from build123d import *

# Parameters (mm, degrees)
SKETCH3_W               = 100
SKETCH3_H               = 210
BOSS_EXTRUDE2_DEPTH     = 5
SKETCH2_W               = 4.8
SKETCH2_H               = 15.2
SKETCH2_W_2             = 5.2
CORTAR_EXTRUIR1_DEPTH   = 2
FILLET1_R               = 2
CUT_EXTRUDE1_DEPTH      = 233.647802483
CUT_EXTRUDE1_DEPTH_BACK = 233.647802483
SKETCH6_R               = 1
CUT_EXTRUDE2_DEPTH      = 3
SKETCH6_4_R             = 1.5
AGUJEROSL298N_DEPTH     = 233.647802483
SKETCH6_6_W             = 68
SKETCH6_6_H             = 35
SKETCH6_6_W_2           = 43
SKETCH6_6_H_2           = 43
SKETCH6_6_H_3           = 20.6
CORTAR_EXTRUIR2_DEPTH   = 2


with BuildPart() as part:
    # Sketch3 → Boss-Extrude2 (new body)
    with BuildSketch(Plane(origin=(0, 0, 0), x_dir=(1, 0, 0), z_dir=(0, 1, 0))):
        with Locations((-50, 105)):
            Rectangle(SKETCH3_W, SKETCH3_H)
    extrude(amount=BOSS_EXTRUDE2_DEPTH)

    # Sketch2 → Cortar-Extruir1 (cut)
    with BuildSketch(Plane(origin=(0, 0, 0), x_dir=(-1, 0, 0), z_dir=(0, -1, 0))):
        with Locations((6, 172.3)):
            Rectangle(SKETCH2_W, SKETCH2_H)
        with Locations((94, 172.3)):
            Rectangle(SKETCH2_W_2, SKETCH2_H)
        with Locations((94, 37.7)):
            Rectangle(SKETCH2_W, SKETCH2_H)
        with Locations((6, 37.7)):
            Rectangle(SKETCH2_W, SKETCH2_H)
    extrude(amount=-CORTAR_EXTRUIR1_DEPTH, mode=Mode.SUBTRACT)

    # Fillet1
    fillet1_edges = [part.edges().sort_by_distance(p)[0] for p in [
        (0, 5, -105),
        (-50, 5, -210),
        (-100, 5, -105),
        (-50, 0, -210),
        (0, 0, -105),
        (-50, 0, 0),
        (-100, 0, -105),
        (-100, 2.5, -210),
        (0, 2.5, -210),
        (-50, 5, 0),
    ]]
    fillet(fillet1_edges, radius=FILLET1_R)

    # Sketch4 → Cut-Extrude1 (cut, two sides: drawn at the far end of the back side and taken through both)
    with BuildSketch(Plane(origin=(0, 5, 0), x_dir=(1, 0, 0), z_dir=(0, 1, 0)).offset(-CUT_EXTRUDE1_DEPTH_BACK)):
        with BuildLine():
            Line((-7.5, 110), (-7.5, 100))
            ThreePointArc((-7.5, 100), (-10, 97.5), (-12.5, 100))
            Line((-12.5, 100), (-12.5, 110))
            ThreePointArc((-12.5, 110), (-10, 112.5), (-7.5, 110))
        make_face()
        with BuildLine():
            Line((-92.5, 110), (-92.5, 100))
            ThreePointArc((-92.5, 100), (-90, 97.5), (-87.5, 100))
            Line((-87.5, 100), (-87.5, 110))
            ThreePointArc((-87.5, 110), (-90, 112.5), (-92.5, 110))
        make_face()
    extrude(amount=CUT_EXTRUDE1_DEPTH + CUT_EXTRUDE1_DEPTH_BACK, mode=Mode.SUBTRACT)

    # Sketch6 → Cut-Extrude2 (cut)
    with BuildSketch(Plane(origin=(0, 5, 0), x_dir=(1, 0, 0), z_dir=(0, 1, 0))):
        with Locations(Location((-80, 202, 0), (0, 0, 270))):
            Circle(SKETCH6_R)
        with Locations(Location((-20, 202, 0), (0, 0, 90))):
            Circle(SKETCH6_R)
        with Locations(Location((-20, 8, 0), (0, 0, 270))):
            Circle(SKETCH6_R)
        with Locations(Location((-80, 8, 0), (0, 0, 90))):
            Circle(SKETCH6_R)
    extrude(amount=-CUT_EXTRUDE2_DEPTH, mode=Mode.SUBTRACT)

    # Sketch6_4 → AgujerosL298N (cut, through all)
    with BuildSketch(Plane(origin=(0, 5, 0), x_dir=(1, 0, 0), z_dir=(0, 1, 0))):
        with Locations(Location((-30.5, 196, 0), (0, 0, 270))):
            Circle(SKETCH6_4_R)
        with Locations(Location((-69.5, 157, 0), (0, 0, 270))):
            Circle(SKETCH6_4_R)
        with Locations(Location((-30.5, 157, 0), (0, 0, 270))):
            Circle(SKETCH6_4_R)
        with Locations(Location((-69.5, 196, 0), (0, 0, 90))):
            Circle(SKETCH6_4_R)
    extrude(amount=-AGUJEROSL298N_DEPTH, mode=Mode.SUBTRACT)

    # Sketch6_6 → Cortar-Extruir2 (cut)
    with BuildSketch(Plane(origin=(0, 5, 0), x_dir=(1, 0, 0), z_dir=(0, 1, 0))):
        with Locations((-50, 29.5)):
            Rectangle(SKETCH6_6_W, SKETCH6_6_H)
        with Locations((-50, 176.5)):
            Rectangle(SKETCH6_6_W_2, SKETCH6_6_H_2)
        with Locations((-50, 70.922705979)):
            Rectangle(SKETCH6_6_W_2, SKETCH6_6_H_3)
        with Locations((-50, 97.904338996)):
            Rectangle(SKETCH6_6_W_2, SKETCH6_6_H_3)
    extrude(amount=-CORTAR_EXTRUIR2_DEPTH, mode=Mode.SUBTRACT)


solid = part.part
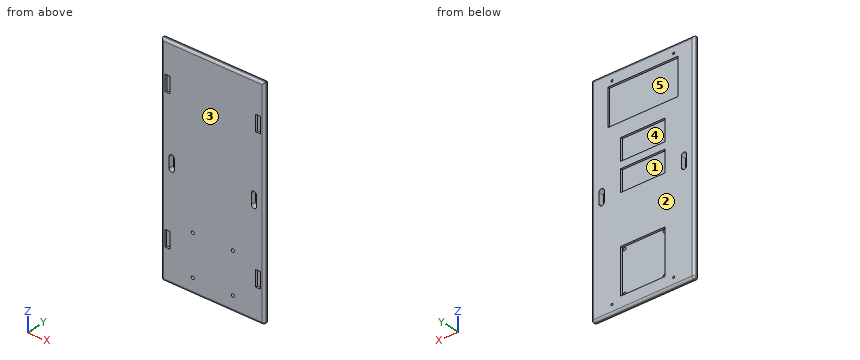
Model file for the job. Use its own axes, mm. Face numbers are marked on the shaded views. A direction names the side the tool comes from. Coordinates: 2 decimals unless noted, no trailing zeros. Write each loop counter-clockwise with the first axis right and the second up, starting at its lowest first coordinate (ties: lowest second). Pieces come first, ordered by that corner, then holes. Notation, with made-up numbers: (-20, -31) -> (-15, -31) arc R19 cw to (-15, -27) -> close; hole circle Ø10 at (-25, 55). An arc over 180 degrees is marked (long way). One line per item, written item: value. Start each with the question number.
1) Slice it at D-D on x = -25.5. Write the cut outline in (y, z), then the cut area to 3 significant figures.
2) Probe probe 1 along Z at (x, y) = (-80, 3.2); probe 2 along X at (y, z) = (2.75, -202); probe 3 along Z at (x, y) = (-69.5, 2.2). List the from-to ranges inside material, lowest first.
3) Flat gauge pins, fed straight in: pin 1 Ø1.8 at (x, z) = (-69.5, -196) entering from -Y; pin 2 Ø17.5 at (x, z) = (-37.5, -30) entering from +Y; pin 3 Ø1.6 at (x, y) = (-6, 1) entering from +Z; pin 4 Ø1 at (x, y) = (-6, 0.5) entering from -Z. Where does each tip first touch, or does it go through?
4) Slice it at B-B on x = -42. Write the cut outline in (y, z).
5) Which spindle directions (+Z, -Z, +X, -X, +Y, -Y) get a long thin tool onto all of the face, cutting with end or side? Do the marked faces 1 and 2. Say none if no direction does.
6) Slice it at C-C on z = -75.5. Write the cut outline in (x, y), then the cut area to 3 significant figures.
7) Slice it at A-A on z = -104.5. Write the cut outline in (x, y).
8) Pull direction X, two halves, no side cores. Call the marked faces 3, 4 and 5: +X half, -X half, draft (parallel to the pull), parting line (faces both ways), or undercut.
Answers follow:
1. outline: (0, -208) arc R2 ccw to (2, -210) -> (3, -210) arc R2 ccw to (5, -208) -> (5, -47) -> (3, -47) -> (3, -12) -> (5, -12) -> (5, -2) arc R2 ccw to (3, 0) -> (2, 0) arc R2 ccw to (0, -2) -> close
1. area: 977 mm2
2. probe 1: -209.99 to -203, -201 to -47, -12 to -9, -7 to -0.01
2. probe 2: -100 to -81, -79 to -21, -19 to 0
2. probe 3: -210 to -197.5, -194.5 to -158.5, -155.5 to 0
3. pin 1: through
3. pin 2: y = 3
3. pin 3: z = -0.01
3. pin 4: z = -209.73
4. outline: (0, -208) arc R2 ccw to (2, -210) -> (3, -210) arc R2 ccw to (5, -208) -> (5, -198) -> (3, -198) -> (3, -155) -> (5, -155) -> (5, -108.2) -> (3, -108.2) -> (3, -87.6) -> (5, -87.6) -> (5, -81.22) -> (3, -81.22) -> (3, -60.62) -> (5, -60.62) -> (5, -47) -> (3, -47) -> (3, -12) -> (5, -12) -> (5, -2) arc R2 ccw to (3, 0) -> (2, 0) arc R2 ccw to (0, -2) -> close
5. face 1: +Y
5. face 2: +Z, -Z, +X, -X, +Y
6. outline: (-100, 2) arc R2 ccw to (-98, 0) -> (-2, 0) arc R2 ccw to (0, 2) -> (0, 3) arc R2 ccw to (-2, 5) -> (-28.5, 5) -> (-28.5, 3) -> (-71.5, 3) -> (-71.5, 5) -> (-98, 5) arc R2 ccw to (-100, 3) -> close
6. area: 411 mm2
7. outline: (-100, 2) arc R2 ccw to (-98, 0) -> (-92.5, 0) -> (-92.5, 5) -> (-98, 5) arc R2 ccw to (-100, 3) -> close; (-87.5, 0) -> (-12.5, 0) -> (-12.5, 5) -> (-28.5, 5) -> (-28.5, 3) -> (-71.5, 3) -> (-71.5, 5) -> (-87.5, 5) -> close; (-7.5, 0) -> (-2, 0) arc R2 ccw to (0, 2) -> (0, 3) arc R2 ccw to (-2, 5) -> (-7.5, 5) -> close
8. face 3: draft
8. face 4: undercut
8. face 5: undercut
